The listing builds one solid part. Answer for the finished solid, in the listing's coordinates (mm). A direction names the side the tool comes from. Coordinates: 2 decimals unless noted, no trailing zeros. Write each loop counter-clockwise with the first axis right and the second up, starting at its lowest first coordinate (ties: lowest second). Pieces come first, ordered by that corner, then holes.
Autodesk Inventor part; units mm, degrees
ref_plane "Work Plane1" through (47, 0, -94) normal (-1, 0, 0) x (0, 0, 1)
ref_plane "YZ Plane" through (0, 0, 0) normal (1, 0, 0) x (0, 1, 0)
ref_plane "XZ Plane" through (0, 0, 0) normal (0, 1, 0) x (-1, 0, 0)
sketch "Sketch3" plane through (0, 0, 0) normal (0, 1, 0) x (-1, 0, 0)
  line L0 (3, 3) -> (-97, 3) construction
  line L1 (-97, 3) -> (-97, 0) construction
  line L2 (-97, 0) -> (3, 0) construction
  line L3 (3, 0) -> (3, 3) construction
  line L4 (-97, 0) -> (-94, 0) construction
  line L5 (-94, 0) -> (-94, -94) construction
  line L6 (-94, -94) -> (-97, -94) construction
  line L7 (-97, -94) -> (-97, 0) construction
  line L8 (-97, -94) -> (3, -94) construction
  line L9 (3, -94) -> (3, -97) construction
  line L10 (3, -97) -> (-97, -97) construction
  line L11 (-97, -97) -> (-97, -94) construction
  line L12 (3, -94) -> (0, -94) construction
  line L13 (0, -94) -> (0, 0) construction
  line L14 (0, 0) -> (3, 0) construction
  line L15 (3, 0) -> (3, -94) construction
  line L16 (0, -94) -> (-94, -94)
  line L17 (-94, -94) -> (-94, 0)
  line L18 (-94, 0) -> (0, 0)
  line L19 (0, 0) -> (0, -94)
  line L20 (3, 3) -> (3, 0) construction
  dimension "d6" = 3
  dimension "d7" = 100
  dimension "d8" = 100
  dimension "d9" = 3
extrude "Extrusion2" add sketch "Sketch3" along normal blind 3
sketch "Sketch4" plane through (0, 3, 0) normal (0, 1, 0) x (1, 0, 0)
  line L0 (94, 94) -> (0, 94)
  line L1 (0, 0) -> (94, 0)
  line L2 (0, 94) -> (5, 94)
  line L3 (5, 94) -> (5, 0)
  line L4 (5, 0) -> (0, 0)
  line L5 (0, 0) -> (0, 94)
  line L6 (94, 0) -> (94, 94)
  line L7 (94, 94) -> (89, 94)
  line L8 (89, 94) -> (89, 0)
  line L9 (89, 0) -> (94, 0)
  line L10 (94, 0) -> (94, 94)
  line L11 (5, 3) -> (89, 3)
  line L12 (89, 3) -> (89, 0)
  line L13 (89, 0) -> (5, 0)
  line L14 (5, 0) -> (5, 3)
  dimension "d12" = 5
  dimension "d13" = 3
extrude "Extrusion3" add sketch "Sketch4" along normal blind 5 contours L6 L1 L8 L0 | L3 L1 L5 L0 | L8 L1 L3 L11
sketch "Sketch6" plane through (94, 0, -94) normal (0, 0, -1) x (-1, 0, 0)
  line L0 (0, 0) -> (94, 0)
  line L1 (89, 8) -> (94, 8)
  line L2 (89, 3) -> (89, 8)
  line L3 (94, 0) -> (94, 8)
  line L4 (0, 0) -> (0, 8)
  point P0 (91.5, 4)
  point P1 (2.5, 4)
  dimension "d28" = 8
  dimension "d29" = 5
  dimension "d30" = 2.5
  dimension "d31" = 4
  dimension "d32" = 2.5
hole "Hole1" at (2.5, 4, -94) at (91.5, 4, -94) direction (0, 0, 1) diameter 2.459 depth 8.8 tip angle 118
fillet "Fillet1" radius 3 2 edges at (89, 5.5, -3) (5, 5.5, -3)
fillet "Fillet2" radius 0.5 2 edges at (5, 5.5, -94) (89, 5.5, -94)
sketch "Sketch7" plane through (0, 0, 0) normal (0, 0, 1) x (1, 0, 0)
  line L0 (0, 0) -> (94, 0)
  line L1 (0, 0) -> (0, 8)
  line L2 (89, 8) -> (5, 8)
  point P0 (19, 4)
  point P1 (47, 4)
  point P2 (75, 4)
  dimension "d40" = 4
  dimension "d57" = 84
  dimension "d58" = 14
  dimension "d59" = 28
  dimension "d60" = 28
hole "Hole2" at (19, 4, 0) at (47, 4, 0) at (75, 4, 0) direction (0, 0, -1) diameter 2.459 depth 3.5 tip angle 118
sketch "Sketch9" plane through (0, 0, -94) normal (-1, 0, 0) x (0, 0, 1)
  line L0 (0, 8) -> (94, 8)
  line L1 (0, 0) -> (94, 0)
  line L2 (0, 0) -> (0, 8)
  point P0 (23.5, 4)
  point P1 (70.5, 4)
  dimension "d51" = 4
  dimension "d52" = 8
  dimension "d53" = 94
  dimension "d54" = 23.5
  dimension "d55" = 47
hole "Hole3" at (0, 4, -70.5) at (0, 4, -23.5) direction (1, 0, 0) diameter 2.459 depth 4 tip angle 118
ref_plane "Work Plane1" through (47, 0, -94) normal (-1, 0, 0) x (0, 0, 1)
mirror "Mirror1" about plane through (47, 0, -94) normal (-1, 0, 0) of "Hole3"
chamfer "Chamfer2" distance 1 angle 45 1 edges at (47, 3, -94)
chamfer "Chamfer3" distance 0.5 angle 45 3 edges at (5, 8, -49.75) (47, 8, -3) (89, 8, -49.75)
ref_plane "Work Plane2" through (47, 0, -94) normal (-1, 0, 0) x (0, 0, 1)
properties part number "LeftPanel" material "Aluminum 6061"
Q1. The part is cut by section B-B, the plane x = 39.5. Write down the section's boundary in (y, z).
Answers below:
outline: (0, -94) - (2, -94) - (3, -93) - (3, -3) - (7.5, -3) - (8, -2.5) - (8, 0) - (0, 0) - close
Q2. Find the intervals of material crossed by probe 1 along X at (y, z) = (4, -88.75); probe 2 along X at (y, z) = (7, -77), in increasing order.
Answers below:
probe 1: x = 0 to 1.27, 3.73 to 5, 89 to 90.27, 92.73 to 94
probe 2: x = 0 to 5, 89 to 94
Q3. Given pin 1 (12 mm diameter, centred on x = 75.5, z = -10.5, fed in from +Y); pin 2 (2 mm diameter, centred on x = 91.5, y = 4, fed in from -Z); pin 3 (2 mm diameter, centred on y = 4, z = -23.5, fed in from +X); pin 4 (1.5 mm diameter, centred on x = 75, y = 4, fed in from -Z), each flat-ended and moving along its own axis, determine where each tip first touches the part or whether it passes through.
Answers below:
pin 1: stops at y = 3
pin 2: stops at z = -85.06
pin 3: stops at x = 89.86
pin 4: passes through
Q4. The part is cut by section A-A, the plane z = -87.5. Write down the section's boundary in (x, y), then the cut area to 3 significant figures.
Answers below:
outline: (0, 0) - (94, 0) - (94, 8) - (89.5, 8) - (89, 7.5) - (89, 3) - (5, 3) - (5, 7.5) - (4.5, 8) - (0, 8) - close; hole circle Ø2.46 at (2.5, 4); hole circle Ø2.46 at (91.5, 4)
area: 322 mm2
Q5. Determine the mould class of faces 4 (the face through (2.45, 2.77, -89.54)), 5 (the face through (91.71, 3.97, -84.59)), 6 (the face through (47, 8, -2)), 7 (the face through (89, 5, -50)) for opening direction Y: released by +Y, released by -Y, zero draft, split by the parting line, or undercut.
Answers below:
face 4: undercut
face 5: undercut
face 6: released by +Y
face 7: zero draft
Q6. Which of the six approach directions +Z, -Z, +X, -X, +Y, -Y give full straight-line access (tool end or side, diameter ignored) to faces 1 (the face through (5, 5, -50)), 2 (the face through (2.03, 3.95, -71.73)), 3 (the face through (91.972, 3.529, -22.364))?
Answers below:
face 1: -Z, +Y
face 2: -X
face 3: +X
Q7. The part is cut by section C-C, the plane z = -76. Write down the section's boundary in (x, y).
Answers below:
outline: (0, 0) - (94, 0) - (94, 8) - (89.5, 8) - (89, 7.5) - (89, 3) - (5, 3) - (5, 7.5) - (4.5, 8) - (0, 8) - close
